Here's how the part is built. I have some questions about the finished solid (model axes, mm). Face numbers are marked on the shaded views. A direction names the side the tool comes from. Give positions to 0.01 mm unless a question says otherwise; leave off trailing zeros. Loops run counter-clockwise (first coordinate to the right, second up) from the corner with the lowest first, then second, coordinate; pieces in that order, holes last. Notation, with made-up numbers: (24.5, 71) - (51.5, 71) arc R27 cw to (51.5, 109) - close; hole circle Ø11 at (-15.75, 56). An arc over 180 degrees is marked (long way). One line per item, written item: value. Start each with the question number.
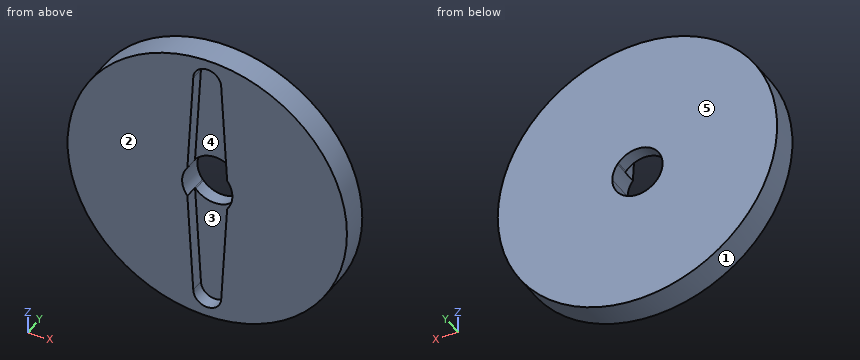
```python
from build123d import *

# Parameters (mm, degrees)
SKETCH1_R           = 20
BOSS_EXTRUDE2_DEPTH = 4
CUT_EXTRUDE2_DEPTH  = 2


with BuildPart() as part:
    # Sketch1 → Boss-Extrude2 (new body)
    with BuildSketch(Plane(origin=(0, 0, 0), x_dir=(1, 0, 0), z_dir=(0, 1, 0))):
        Circle(SKETCH1_R)
        with BuildLine():
            ThreePointArc((3.6, 0), (3.406815835, 1.163445687), (2.847996741, 2.202025105))
            Line((2.847996741, 2.202025105), (1.999997781, 16.602979385))
            ThreePointArc((1.999997781, 16.602979385), (0, 18.6), (-1.999997781, 16.602979385))
            Line((-1.999997781, 16.602979385), (-2.847996741, 2.202025105))
            ThreePointArc((-2.847996741, 2.202025105), (-3.6, 0), (-2.847996741, -2.202025105))
            Line((-2.847996741, -2.202025105), (-1.999997781, -16.602979385))
            ThreePointArc((-1.999997781, -16.602979385), (0, -18.6), (1.999997781, -16.602979385))
            Line((1.999997781, -16.602979385), (2.847996741, -2.202025105))
            ThreePointArc((2.847996741, -2.202025105), (3.406815835, -1.163445687), (3.6, 0))
        make_face(mode=Mode.SUBTRACT)
        with BuildLine():
            ThreePointArc((2.739990437, -2.335048694), (0, -3.6), (-2.739990437, -2.335048694))
            Line((-2.739990437, -2.335048694), (-1.9, -16.6))
            ThreePointArc((-1.9, -16.6), (0, -18.5), (1.9, -16.6))
            Line((1.9, -16.6), (2.739990437, -2.335048694))
        make_face()
        with BuildLine():
            Line((-1.9, 16.6), (-2.739990437, 2.335048694))
            ThreePointArc((-2.739990437, 2.335048694), (0, 3.6), (2.739990437, 2.335048694))
            Line((2.739990437, 2.335048694), (1.9, 16.6))
            ThreePointArc((1.9, 16.6), (0, 18.5), (-1.9, 16.6))
        make_face()
        with BuildLine():
            Line((-1.9, -16.6), (-2.739990437, -2.335048694))
            ThreePointArc((-2.739990437, -2.335048694), (-2.794785143, -2.269179589), (-2.847996741, -2.202025105))
            Line((-2.847996741, -2.202025105), (-1.999997781, -16.602979385))
            ThreePointArc((-1.999997781, -16.602979385), (0, -18.6), (1.999997781, -16.602979385))
            Line((1.999997781, -16.602979385), (2.847996741, -2.202025105))
            ThreePointArc((2.847996741, -2.202025105), (2.794785143, -2.269179589), (2.739990437, -2.335048694))
            Line((2.739990437, -2.335048694), (1.9, -16.6))
            ThreePointArc((1.9, -16.6), (0, -18.5), (-1.9, -16.6))
        make_face()
        with BuildLine():
            ThreePointArc((-2.847996741, 2.202025105), (-2.794785143, 2.269179589), (-2.739990437, 2.335048694))
            Line((-2.739990437, 2.335048694), (-1.9, 16.6))
            ThreePointArc((-1.9, 16.6), (0, 18.5), (1.9, 16.6))
            Line((1.9, 16.6), (2.739990437, 2.335048694))
            ThreePointArc((2.739990437, 2.335048694), (2.794785143, 2.269179589), (2.847996741, 2.202025105))
            Line((2.847996741, 2.202025105), (1.999997781, 16.602979385))
            ThreePointArc((1.999997781, 16.602979385), (0, 18.6), (-1.999997781, 16.602979385))
            Line((-1.999997781, 16.602979385), (-2.847996741, 2.202025105))
        make_face()
    extrude(amount=BOSS_EXTRUDE2_DEPTH)

    # Sketch1_6 → Cut-Extrude2 (cut)
    with BuildSketch(Plane(origin=(0, 0, 0), x_dir=(1, 0, 0), z_dir=(0, 1, 0))):
        with BuildLine():
            Line((-1.9, -16.6), (-2.739990437, -2.335048694))
            ThreePointArc((-2.739990437, -2.335048694), (-2.794785143, -2.269179589), (-2.847996741, -2.202025105))
            Line((-2.847996741, -2.202025105), (-1.999997781, -16.602979385))
            ThreePointArc((-1.999997781, -16.602979385), (0, -18.6), (1.999997781, -16.602979385))
            Line((1.999997781, -16.602979385), (2.847996741, -2.202025105))
            ThreePointArc((2.847996741, -2.202025105), (2.794785143, -2.269179589), (2.739990437, -2.335048694))
            Line((2.739990437, -2.335048694), (1.9, -16.6))
            ThreePointArc((1.9, -16.6), (0, -18.5), (-1.9, -16.6))
        make_face()
        with BuildLine():
            ThreePointArc((2.739990437, -2.335048694), (0, -3.6), (-2.739990437, -2.335048694))
            Line((-2.739990437, -2.335048694), (-1.9, -16.6))
            ThreePointArc((-1.9, -16.6), (0, -18.5), (1.9, -16.6))
            Line((1.9, -16.6), (2.739990437, -2.335048694))
        make_face()
        with BuildLine():
            Line((-1.9, 16.6), (-2.739990437, 2.335048694))
            ThreePointArc((-2.739990437, 2.335048694), (0, 3.6), (2.739990437, 2.335048694))
            Line((2.739990437, 2.335048694), (1.9, 16.6))
            ThreePointArc((1.9, 16.6), (0, 18.5), (-1.9, 16.6))
        make_face()
        with BuildLine():
            ThreePointArc((-2.847996741, 2.202025105), (-2.794785143, 2.269179589), (-2.739990437, 2.335048694))
            Line((-2.739990437, 2.335048694), (-1.9, 16.6))
            ThreePointArc((-1.9, 16.6), (0, 18.5), (1.9, 16.6))
            Line((1.9, 16.6), (2.739990437, 2.335048694))
            ThreePointArc((2.739990437, 2.335048694), (2.794785143, 2.269179589), (2.847996741, 2.202025105))
            Line((2.847996741, 2.202025105), (1.999997781, 16.602979385))
            ThreePointArc((1.999997781, 16.602979385), (0, 18.6), (-1.999997781, 16.602979385))
            Line((-1.999997781, 16.602979385), (-2.847996741, 2.202025105))
        make_face()
    extrude(amount=CUT_EXTRUDE2_DEPTH, mode=Mode.SUBTRACT)


solid = part.part
```
(1) If we section it at B-B on x = 0: List the corners of the cut face in (y, z) for me, plus the area to 3 significant figures.
(2) Will these pins go through, and if not, where does the flat tip stop? pin 1 (1 mm diameter, centred on y = 0.5, z = -15, fed in from -X) (3 decimals); pin 2 (2 mm diameter, centred on x = 9.5, y = 3.5, fed in from +Z); pin 3 (3 mm diameter, centred on x = 0.5, z = 11, fed in from -Y).
(3) If we mould it in two halves opening along Z, with no side actions, what happens to the marked faces 1, 2 and 3? For each: pulls with the +Z half, pulls with the -Z half, needs draft (parallel to the pull), parting line crosses it, or undercut.
(4) Please list where these lines run through material, in increasing order: probe 1 along X at (y, z) = (1.3, 2.5); probe 2 along Z at (x, y) = (-0.5, 0.9); probe 3 along Z at (x, y) = (1, 2.35). Write a range as from..to.
(5) If we section it at C-C on z = -18: List the corners of the cut face in (x, y) for me, plus the area to 3 significant figures.
(6) If we section it at D-D on x = -12: List the corners of the cut face in (y, z) for me, plus the area to 3 significant figures.
(7) For the marked faces 4 and 5, which set-ups out of +Z, -Z, +X, -X, +Y, -Y let a thin tool reach every point of the face, with its end or its side?
(8) If we section it at A-A on y = 1.15: List the corners of the cut face in (x, z) for me.
Found:
1. outline: (0, -20) - (4, -20) - (4, -3.6) - (2, -3.6) - (2, -18.6) - (0, -18.6) - close; (0, 18.6) - (2, 18.6) - (2, 3.6) - (4, 3.6) - (4, 20) - (0, 20) - close
1. area: 71.2 mm^2
2. pin 1: x = -13.775
2. pin 2: z = 18.1
2. pin 3: y = 2
3. face 1: parting line crosses it
3. face 2: needs draft
3. face 3: undercut
4. probe 1: -19.84..-2.83, 2.83..19.84
4. probe 2: -19.99..-18.54, 18.54..19.99
4. probe 3: -19.97..-3.46, 3.46..19.97
5. outline: (-8.72, 0) - (-1.43, 0) - (-1.43, 2) - (1.43, 2) - (1.43, 0) - (8.72, 0) - (8.72, 4) - (-8.72, 4) - close
5. area: 64.0 mm^2
6. outline: (0, -16) - (4, -16) - (4, 16) - (0, 16) - close
6. area: 128 mm^2
7. face 4: -Y
7. face 5: +Z, -Z, +X, -X, +Y
8. outline: circle Ø40 at (0, 0); hole (-2.85, -2.2) - (-2, -16.6) arc R2 ccw to (2, -16.6) - (2.85, -2.2) arc R3.6 ccw to (2.85, 2.2) - (2, 16.6) arc R2 ccw to (-2, 16.6) - (-2.85, 2.2) arc R3.6 ccw to start
